Build history of the part. All positions in model axes, mm. Face numbers are marked on the shaded views. Coordinates: 2 decimals unless noted, no trailing zeros. Order: outer loops, then holes, each group sorted by start corner. A loop starts at its lowest first (then second) coordinate and runs counter-clockwise, first axis right, second up. Notation, with made-up numbers: M 74,-31 L 126,-31 A12 ccw 126,-25 Z; hole C 47,67.5 d5. An arc over 180 degrees is marked long. Write item = value, one per line. Start each with the question number.
Q1. Pull direction X, two halves, no side cores. Call the marked faces 1 and 2: released by +X, released by -X, zero draft, split by the parting line, or undercut.
Q2. Drill centre lines: probe 1 along Z at (x, y) = (23.5, 7.5); probe 2 along X at (y, z) = (-0.5, 2.4); probe 3 along X at (y, z) = (13, 2.2). Where is each one in solid material? Low to high.
Q3. Band-saw the part on D-D on y = -23.5. Write the cut outline in (x, z).
Q4. Pin check, flat tips, straight feed: P1, Ø12, axis at x = -4, y = 18.5, coming from the -Z side; P2, Ø17.5, axis at x = -2, y = 8.5, coming from the +Z side; P3, Ø1.5, axis at x = 14, z = 1.5, coming from the -Y side. Stop position of each tip, or through.
Q5. Band-saw the part on C-C on z = 0.6. Write the cut outline in (x, y).
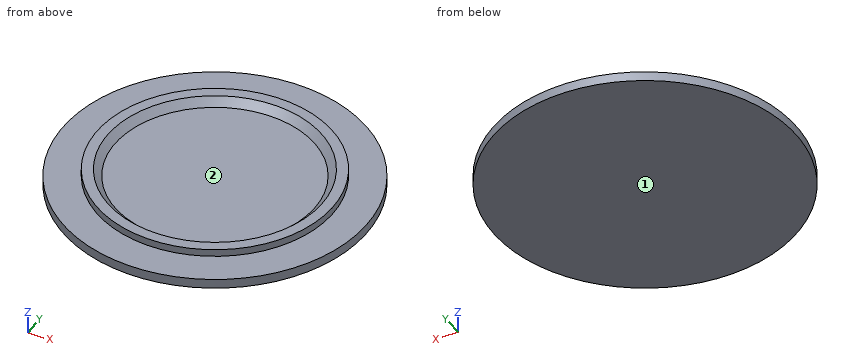
```python
from build123d import *

# Parameters (mm, degrees)
F0_R     = 26.9
F0_R_2   = 20.9
F1_DEPTH = 1.7
F2_DEPTH = 3
F3_R     = 19
F4_DEPTH = 1.3
F5_SIZE  = 1.29999


# Not quite as in the source:
# - a fillet or chamfer is up to 0.001 mm smaller than in the source, because OpenCascade refuses the exact size


with BuildPart() as f1:
    # F0 (on Top) → F1 (new body)
    with BuildSketch(Plane.XY):
        Circle(F0_R)
        Circle(F0_R_2, mode=Mode.SUBTRACT)
    extrude(amount=F1_DEPTH)

    # F0 (on Top) → F2 (join)
    with BuildSketch(Plane.XY):
        Circle(F0_R_2)
    extrude(amount=F2_DEPTH)

    # F3 (on face) → F4 (cut)
    with BuildSketch(Plane.XY.offset(3)):
        Circle(F3_R)
    extrude(amount=-F4_DEPTH, mode=Mode.SUBTRACT)

    # F5 (size 1.3 in the source; OpenCascade refuses exactly that, so slightly less here)
    f5_edges = [f1.edges().sort_by_distance(p)[0] for p in [
        (-19, 0, 1.7),
    ]]
    chamfer(f5_edges, length=F5_SIZE)


solid = f1.part
```
Recorded:
q1.face_1 = zero draft
q1.face_2 = undercut
q2.probe_1 = 0 to 1.7
q2.probe_2 = -20.89 to -18.39, 18.39 to 20.89
q2.probe_3 = -16.36 to -12.74, 12.74 to 16.36
q3.outline = M -13.09,0 L 13.09,0 L 13.09,1.7 L -13.09,1.7 Z
q4.P1 = 0
q4.P2 = 1.7
q4.P3 = -23.41
q5.outline = C 0,0 d53.8
